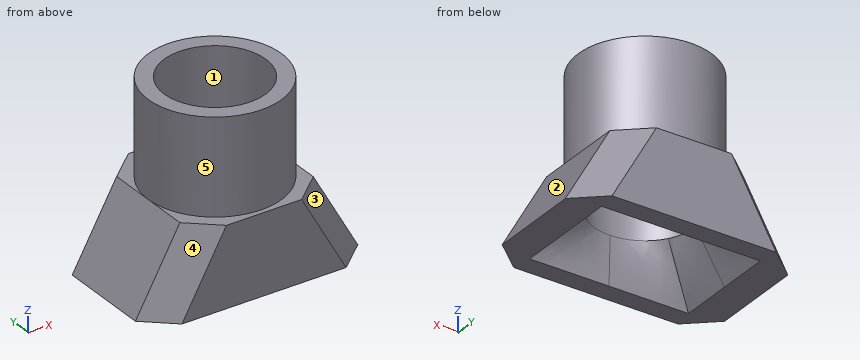
Autodesk Fusion 360 part; units mm, degrees
sketch "草图1" plane through (0, 0, 0) normal (0, 1, 0) x (1, 0, 0)
  line L0 (0, 0) -> (70, 0)
  line L1 (70, 0) -> (70, -55)
  line L2 (70, -55) -> (0, -55)
  line L3 (0, -55) -> (0, 0)
  dimension "d1" = 70
  dimension "d2" = 55
extrude "拉伸1" add sketch "草图1" along normal blind 45
sketch "草图2" plane through (0, 0, 55) normal (0, 0, 1) x (-1, 0, 0)
  line L0 (0, 0) -> (-70, 0)
  line L1 (-70, 0) -> (-70, -45)
  line L2 (-70, -45) -> (0, -45)
  line L3 (0, -45) -> (0, 0)
  line L4 (-35, -45) -> (-35, -22.5)
  circle A0 centre (-35, -22.5) radius 16
  circle A1 centre (-35, -22.5) radius 21
  dimension "d5" = 22.5
  dimension "d6" = 32
  dimension "d12" = 42
extrude "拉伸2" cut sketch "草图2" against normal blind 40 contours A0
sketch "草图3" plane through (0, 0, 0) normal (0, 0, -1) x (1, 0, 0)
  line L0 (70, 0) -> (0, 0)
  line L1 (0, 0) -> (0, -45)
  line L2 (0, -45) -> (70, -45)
  line L3 (70, -45) -> (70, 0)
  line L4 (35, 0) -> (35, -22.5)
  line L5 (60, -39) -> (10, -39)
  line L6 (10, -39) -> (10, -6)
  line L7 (10, -6) -> (60, -6)
  line L8 (60, -6) -> (60, -39)
  line L9 (60, -39) -> (10, -6) construction
  line L10 (10, -39) -> (60, -6) construction
  point P0 (35, -22.5)
  dimension "d9" = 22.5
  dimension "d10" = 50
  dimension "d11" = 33
sketch "草图4" plane through (0, 0, 15) normal (0, 0, 1) x (-1, 0, 0)
  circle A0 centre (-35, -22.5) radius 16
loft "放样1" cut profiles "草图4", "草图3" section 1 section 2 contours L5 L6 L7 L8
extrude "拉伸4" cut sketch "草图2" against normal blind 30 contours L0 L1 L2 L3
sketch "草图5" plane through (0, 0, 25) normal (0, 0, 1) x (-1, 0, 0)
  circle A0 centre (-35, -22.5) radius 21
  line L0 (0, -45) -> (0, 0)
  line L1 (0, 0) -> (-70, 0)
  line L2 (-70, 0) -> (-70, -45)
  line L3 (-70, -45) -> (0, -45)
  circle A1 centre (-35, -22.5) radius 21
sketch "草图6" plane through (0, 45, 0) normal (0, 1, 0) x (-1, 0, 0)
  line L0 (0, 25) -> (-70, 25)
  line L1 (-70, 25) -> (-70, 0)
  line L2 (-70, 0) -> (0, 0)
  line L3 (0, 0) -> (0, 25)
  line L4 (-35, 25) -> (-56, 25)
  line L5 (-56, 25) -> (-70, 0)
  line L6 (-35, 25) -> (-14, 25)
  line L7 (-14, 25) -> (0, 0)
  dimension "d17" = 21
  dimension "d18" = 21
extrude "拉伸5" cut sketch "草图6" against normal blind 45 contours L0 L3 L7 | L0 L1 L5
chamfer "倒角1" distance 8 angle 45 4 edges at (7, 45, 12.5) (7, 0, 12.5) (63, 45, 12.5) (63, 0, 12.5)
extrude "拉伸3" [suppressed]
Could you check a few things on this model? Use its own coordinates, in mm. Face numbers are marked on the shaded views. A direction names the side the tool comes from. Round coordinates to 2 decimals unless told otherwise and drop trailing zeros. Loops run counter-clockwise (first coordinate to the right, second up) from the corner with the lowest first, then second, coordinate; pieces in that order, holes last.
Q1. On a 3-axis mill with a long thin cutter (end or side, diameter ignored), from which of +Z, -Z, +X, -X, +Y, -Y can I reach the whole of each face in a straight line? I mean the marked faces 4 and 5. Say none if no direction works.
Q2. I want a section at C-C (x = 8). Write out the boundary of the cut face in (y, z).
Q3. I want a section at A-A (z = 41). Write out the boundary of the cut face in (x, y), and give its area (3 significant figures).
Q4. For P1, Ø5, axis at y = 28, z = 24, coming from the +X side; P2, Ø4, axis at y = 21, z = 31.5, coming from the +X side; P3, Ø1, axis at y = 5, z = 42, coming from the +X side, each with a flat end and sliding along its axis, tell me the tip position at first contact or that it passes through.
Q5. I want a section at B-B (y = 40.5). Write out the boundary of the cut face in (x, z), and give its area (3 significant figures).
Q6. Thinking about a two-plate mould opening in Y: for the marked faces 1, 2 and 3, which applies, pulls with the +Y half, pulls with the -Y half, needs draft (parallel to the pull), parting line crosses it, or undercut?
Q7. Please list where these lines run through material, in increasing order: L1, parallel to Y at x = 35, z = 40; L2, parallel to X at y = 22, z = 37; L3, parallel to X at y = 12.5, z = 17.
Q8. I want a section at D-D (z = 16). Write out the boundary of the cut face in (x, y).
Answer below:
1. face 4: +Z, -X, -Y
1. face 5: +Z
2. outline: (1.02, 0) - (43.98, 0) - (37, 14.29) - (8, 14.29) - close
3. outline: circle Ø42 at (35, 22.5); hole circle Ø32 at (35, 22.5)
3. area: 581 mm2
4. P1: stops at x = 57.96
4. P2: stops at x = 56
4. P3: stops at x = 47.33
5. outline: (4.01, 0) - (65.99, 0) - (51.99, 25) - (45.82, 25) - (45.82, 55) - (24.18, 55) - (24.18, 25) - (18.01, 25) - close
5. area: 1,850 mm2
6. face 1: undercut
6. face 2: needs draft
6. face 3: pulls with the -Y half
7. L1: y = 1.5 to 6.5, 38.5 to 43.5
7. L2: x = 14.01 to 19.01, 50.99 to 55.99
7. L3: x = 9.52 to 22.51, 47.49 to 60.48
8. outline: (8.96, 8) - (18.13, 0) - (51.87, 0) - (61.04, 8) - (61.04, 37) - (51.87, 45) - (18.13, 45) - (8.96, 37) - close; hole circle Ø32 at (35, 22.5)
